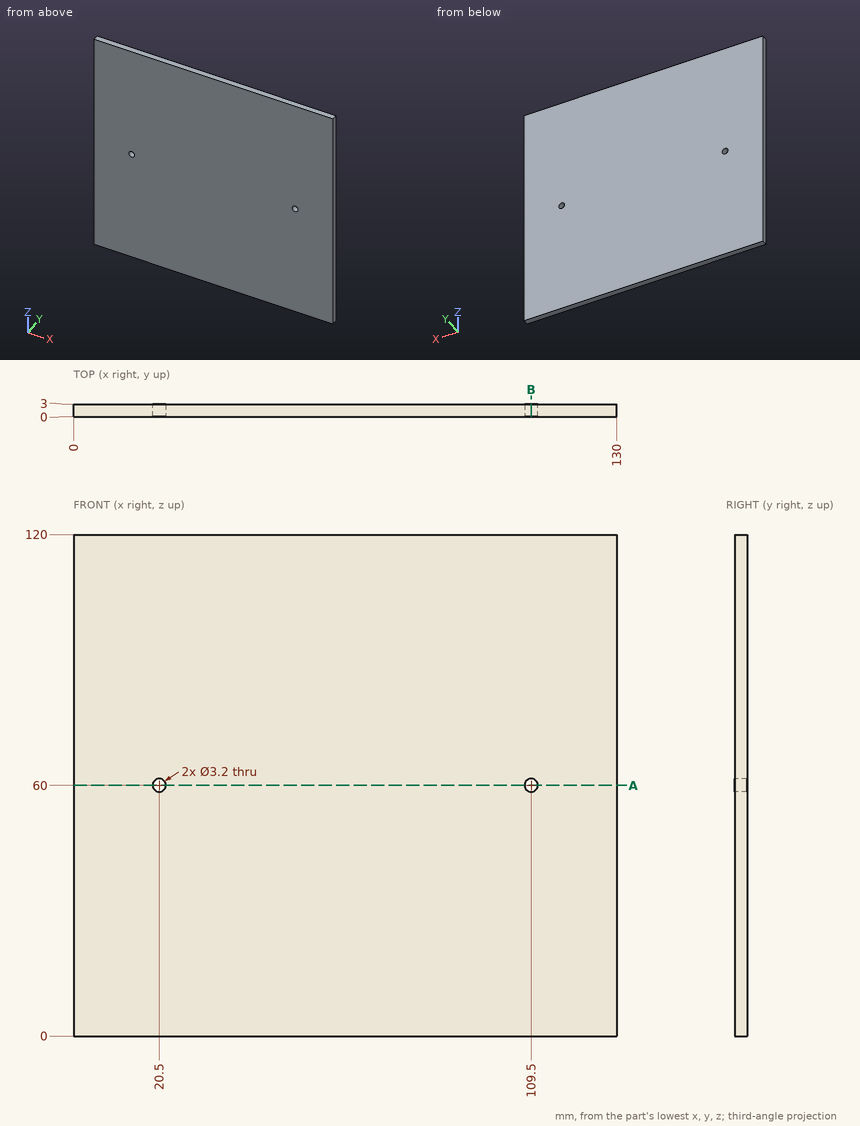
Input: dimensioned drawing with shaded views. Units: mm. Origin: part minimum x, y, z. Give positions to 0.01 mm unless a question says otherwise; leave off trailing zeros. Loops run counter-clockwise (first coordinate to the right, second up) from the corner with the lowest first, then second, coordinate; pieces in that order, holes last. Notation, with made-up numbers: (39.25, 75) -> (53.25, 75) arc R17 ccw to (53.25, 92) -> close; hole circle Ø4 at (-11, 88.25). An arc over 180 degrees is marked (long way). Use a Markdown table: item, result. Add a question column.
1) Line query: line 1 along Z through (x, y) = (109.5, 0.8). Output: solid intervals per line, ascending. Write a range as [from, to].
2) First-contact query: pin 1 (1.9 mm diameter, centred on x = 20.5, z = 60, fed in from -Y). Flat tip, straight axial feed; report the tip coordinate or a pass-through.
3) Section query B-B, the plane x = 109.5. Return the cut outline in (y, z), then the cut area to 3 significant figures.
4) Section query A-A, the plane z = 60. Return the cut outline in (x, y), then the cut area to 3 significant figures.
Numbers:
| question | item | result |
|---|---|---|
| 1 | line 1 | z = [0, 58.4], [61.6, 120] |
| 2 | pin 1 | passes through |
| 3 | outline | (0, 0) -> (3, 0) -> (3, 58.4) -> (0, 58.4) -> close; (0, 61.6) -> (3, 61.6) -> (3, 120) -> (0, 120) -> close |
| 3 | area | 350 mm2 |
| 4 | outline | (0, 0) -> (18.9, 0) -> (18.9, 3) -> (0, 3) -> close; (22.1, 0) -> (107.9, 0) -> (107.9, 3) -> (22.1, 3) -> close; (111.1, 0) -> (130, 0) -> (130, 3) -> (111.1, 3) -> close |
| 4 | area | 371 mm2 |
